```python
from build123d import *

# Parameters (mm, degrees)
EXTRUDE_1_DEPTH     = 1.5
SKETCH_2_R          = 3.025074469
CUT_EXTRUDE_1_DEPTH = 16.272715323


with BuildPart() as part:
    # 草图1 → 凸台-拉伸1 (new body)
    with BuildSketch(Plane.XY):
        Polygon((11.489270357, 0), (5.744635178, 9.95), (-5.744635178, 9.95), (-11.489270357, 0), (-5.744635178, -9.95), (5.744635178, -9.95), align=None)
    extrude(amount=EXTRUDE_1_DEPTH)

    # 草图2 → 切除-拉伸1 (cut, through all)
    with BuildSketch(Plane.XY.offset(1.5)):
        with Locations((-9.5, 0)):
            Circle(SKETCH_2_R)
        with Locations((-4.75, 8.227241336)):
            Circle(SKETCH_2_R)
        with Locations((4.75, 8.227241336)):
            Circle(SKETCH_2_R)
        with Locations((9.5, 0)):
            Circle(SKETCH_2_R)
        with Locations((4.75, -8.227241336)):
            Circle(SKETCH_2_R)
        with Locations((-4.75, -8.227241336)):
            Circle(SKETCH_2_R)
    extrude(amount=-CUT_EXTRUDE_1_DEPTH, mode=Mode.SUBTRACT)

    # 草图4 → 旋转-薄壁2 (revolve)
    with BuildSketch(Plane(origin=(0, 0, 0), x_dir=(0, 0, -1), z_dir=(1, 0, 0)), mode=Mode.PRIVATE) as revolve_2_sk:
        with BuildLine():
            Line((0, 0), (3.62, 0))
            ThreePointArc((3.62, 0), (2.559726548, 2.559726548), (0, 3.62))
            Line((0, 3.62), (0, 3.52))
            ThreePointArc((0, 3.52), (2.453405796, 2.52412361), (3.518579259, 0.1))
            Line((3.518579259, 0.1), (0, 0.1))
            Line((0, 0.1), (0, 0))
        make_face()
    revolve(revolve_2_sk.sketch.rotate(Axis((0, 0, 0), (0, 0, -1)), 90), axis=Axis((0, 0, 0), (0, 0, -1)))


solid = part.part
```
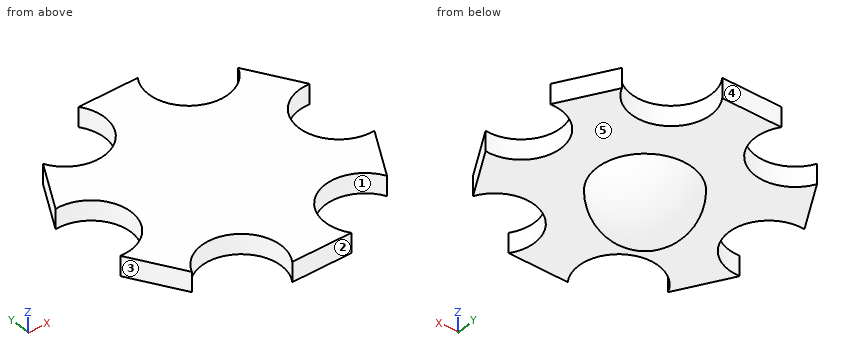
CAD build for the part. Positions are in the model's coordinates, mm. Face numbers are marked on the shaded views. A direction names the side the tool comes from. Round coordinates to 2 decimals unless told otherwise and drop trailing zeros. Order: outer loops, then holes, each group sorted by start corner. A loop starts at its lowest first (then second) coordinate and runs counter-clockwise, first axis right, second up. Notation, with made-up numbers: (78.25, -18) -> (84.25, -18) arc R23 ccw to (84.25, 3) -> close; hole circle Ø8 at (35, 20). An arc over 180 degrees is marked (long way). One line per question, with ' | ' between items.
Q1. Drop flat-ended pins along their axis: pin 1 (5 mm diameter, centred on x = 4.75, y = 8.23, fed in from -Z); pin 2 (9.5 mm diameter, centred on x = -9.5, y = 0, fed in from -Z); pin 3 (3 mm diameter, centred on y = -1.5, z = -2.5, fed in from +X); pin 4 (1.5 mm diameter, centred on y = 5, z = -0.5, fed in from +X). Give the stop position or say it passes through.
Completed:
pin 1: passes through | pin 2: stops at z = 0 | pin 3: stops at x = 3.33 | pin 4: stops at x = 8.93
Q2. Slice it at B-B (x = 9.5). Write the cut outline in (y, z).
Completed:
outline: (-3.45, 0) -> (-3.03, 0) -> (-3.03, 1.5) -> (-3.45, 1.5) -> close; (3.03, 0) -> (3.45, 0) -> (3.45, 1.5) -> (3.03, 1.5) -> close
Q3. Probe probe 1 along Z at (x, y) = (5.5, -1.25); probe 2 along X at (y, z) = (0, 0.4); probe 3 along Y at (x, z) = (4.75, 0.4). List the from-to ranges inside material, lowest first.
Completed:
probe 1: z = 0 to 1.5 | probe 2: x = -6.47 to 6.47 | probe 3: y = -5.2 to 5.2
Q4. Slice it at A-A (y = -6.5). Write the cut outline in (x, z), then the cut area to 3 significant figures.
Completed:
outline: (-7.74, 0) -> (-7.23, 0) -> (-7.23, 1.5) -> (-7.74, 1.5) -> close; (-2.27, 0) -> (2.27, 0) -> (2.27, 1.5) -> (-2.27, 1.5) -> close; (7.23, 0) -> (7.74, 0) -> (7.74, 1.5) -> (7.23, 1.5) -> close | area: 8.31 mm^2
Q5. Which spindle directions (+Z, -Z, +X, -X, +Y, -Y) get a long thin tool onto all of the face, cutting with end or side? Do the marked faces 4 and 5. Say none if no direction does.
Completed:
face 4: +Z, -Z, +X, -X, +Y | face 5: -Z
Q6. Two-plate mould, pull along X, no slides. Class the marked faces 1, 2 and 3: released by +X, released by -X, zero draft, split by the parting line, or undercut.
Completed:
face 1: undercut | face 2: zero draft | face 3: released by -X
Q7. Slice it at D-D (x = -0.5). Write the cut outline in (y, z), then the cut area to 3 significant figures.
Completed:
outline: (-9.95, 0) -> (-3.59, 0) arc R3.59 ccw to (3.59, 0) -> (9.95, 0) -> (9.95, 1.5) -> (-9.95, 1.5) -> close; hole (-3.48, 0) arc R3.48 ccw to (3.48, 0) -> close | area: 31.0 mm^2
